Autodesk Inventor part; units mm, degrees
ref_plane "YZ Plane" through (0, 0, 0) normal (1, 0, 0) x (0, 1, 0)
ref_plane "XZ Plane" through (0, 0, 0) normal (0, 1, 0) x (-1, 0, 0)
ref_plane "XY Plane" through (0, 0, 0) normal (0, 0, 1) x (1, 0, 0)
sketch "Sketch1" plane through (0, 0, 0) normal (0, 1, 0) x (-1, 0, 0)
  line L0 (2.0728, 0) -> (87.1628, 0)
  line L1 (87.1628, 0) -> (87.1628, -50.165)
  line L2 (87.1628, -50.165) -> (2.0728, -50.165)
  line L3 (2.0728, -50.165) -> (2.0728, 0)
  line L4 (87.1628, -50.165) -> (2.0728, 0)
  point P0 (0, 0)
  dimension "d0" = 85.09
  dimension "d1" = 50.165
extrude "Extrusion1" add sketch "Sketch1" along normal blind 3.175 contours L0 L1 L4
sketch "Sketch2" plane through (0, 3.175, 0) normal (0, 1, 0) x (1, 0, 0)
  line L0 (-87.1628, 0) -> (-2.0728, 0)
  line L1 (-87.1628, 0) -> (-90.3378, 0)
  line L2 (-90.3378, 0) -> (-90.3378, 50.165)
  line L3 (-90.3378, 50.165) -> (-87.1628, 50.165)
  line L4 (-87.1628, 50.165) -> (-87.1628, 0)
  line L5 (-87.1628, 0) -> (-2.0728, 0)
  line L6 (-2.0728, 0) -> (-2.0728, -3.175)
  line L7 (-2.0728, -3.175) -> (-87.1628, -3.175)
  line L8 (-87.1628, -3.175) -> (-87.1628, 0)
  line L9 (-90.3378, 0) -> (-87.1628, 0)
  line L10 (-87.1628, 0) -> (-87.1628, -3.175)
  line L11 (-87.1628, -3.175) -> (-90.3378, -3.175)
  line L12 (-90.3378, -3.175) -> (-90.3378, 0)
  point P0 (0, 0)
  dimension "d4" = 3.175
  dimension "d5" = 3.175
extrude "Extrusion2" add sketch "Sketch2" along normal blind 34.7726 contours L1 L2 L3 L4 | L0 L6 L7 L8
sketch "Sketch3" plane through (0, 37.9476, 0) normal (0, 1, 0) x (1, 0, 0)
  line L0 (-87.1628, 0) -> (-90.3378, 0)
  line L1 (-90.3378, 0) -> (-90.3378, -3.175)
  line L2 (-90.3378, -3.175) -> (-87.1628, -3.175)
  line L3 (-87.1628, -3.175) -> (-87.1628, 0)
  point P0 (0, 0)
  dimension "d8" = 3.175
extrude "Extrusion3" add sketch "Sketch3" against normal blind 34.7726
sketch "Sketch4" plane through (0, 3.175, 0) normal (0, -1, 0) x (1, 0, 0)
  line L0 (-87.1628, 0) -> (-2.0728, 0)
  line L1 (-2.0728, 3.175) -> (-2.0728, 0)
  line L2 (-2.0728, 3.175) -> (-90.3378, 3.175)
  line L3 (-90.3378, -50.165) -> (-90.3378, 3.175)
  line L4 (-87.1628, -50.165) -> (-90.3378, -50.165)
  line L5 (-87.1628, -50.165) -> (-87.1628, 0)
  point P0 (0, 0)
extrude "Extrusion4" add sketch "Sketch4" along normal blind 3.175
fillet "Fillet1" radius 3.175 2 edges at (-46.2053, 0, 3.175) (-90.3378, 0, -23.495)
sketch "Sketch5" plane through (0, 0, 0) normal (0, -1, 0) x (1, 0, 0)
  line L0 (-87.0358, -0.127) -> (-90.3378, -0.127)
  line L1 (-90.3378, -0.127) -> (-90.3378, 3.175)
  line L2 (-90.3378, 3.175) -> (-87.0358, 3.175)
  line L3 (-87.0358, 3.175) -> (-87.0358, -0.127)
  line L4 (-90.3378, 0) -> (-90.3378, -50.165)
  line L5 (-2.0728, 3.175) -> (-87.1628, 3.175)
  point P0 (0, 0)
  dimension "d22" = 3.302
  dimension "d23" = 3.302
  dimension "d24" = 0
  dimension "d25" = 0
extrude "Extrusion5" cut sketch "Sketch5" against normal blind 127
chamfer "Chamfer4" distance 3.175 angle 45 4 edges at (-2.0728, 37.9476, 1.5875) (-88.7503, 37.9476, -50.165) (-88.7503, 37.9476, -0.127) (-87.0358, 37.9476, 1.5875)
sketch "Sketch6" plane through (-87.1628, 3.175, -0.127) normal (1, 0, 0) x (0, 0, -1)
  line L0 (50.038, 0) -> (50.038, 31.5976)
  line L1 (3.175, 34.7726) -> (46.863, 34.7726)
  circle A0 centre (38.608, 25.3746) radius 2.54
  circle A1 centre (38.608, 12.6746) radius 2.54
  circle A2 centre (25.908, 25.3746) radius 2.54
  circle A3 centre (25.908, 12.6746) radius 2.54
  circle A4 centre (13.208, 25.3746) radius 2.54
  circle A5 centre (13.208, 12.6746) radius 2.54
  point P0 (-0.127, -3.175)
  dimension "d43" = 25.4
  dimension "d32" = 5.08
  dimension "d34" = 11.43
  dimension "d35" = 9.398
  dimension "d36" = 5.08
  dimension "d37" = 12.7
  dimension "d40" = 12.7
extrude "Extrusion6" cut sketch "Sketch6" against normal blind 127
sketch "Sketch7" plane through (-2.0728, 3.175, 0) normal (0, 0, -1) x (-1, 0, 0)
  line L0 (3.175, 34.7726) -> (81.788, 34.7726)
  line L1 (84.963, 0) -> (0, 0)
  line L2 (84.963, 0) -> (84.963, 31.5976)
  circle A0 centre (78.613, 25.8826) radius 2.54
  circle A1 centre (47.752, 25.8826) radius 2.54
  circle A2 centre (16.891, 25.8826) radius 2.54
  circle A3 centre (78.613, 11.6586) radius 2.54
  circle A4 centre (47.752, 11.6586) radius 2.54
  circle A5 centre (16.891, 11.6586) radius 2.54
  point P0 (-2.0728, -3.175)
  dimension "d48" = 5.08
  dimension "d49" = 6.35
  dimension "d50" = 8.89
  dimension "d53" = 30.861
  dimension "d56" = 14.224
extrude "Extrusion7" cut sketch "Sketch7" against normal blind 127
sketch "Sketch8" plane through (0, 3.175, 0) normal (0, 1, 0) x (1, 0, 0)
  line L0 (-87.0358, 0) -> (-2.0728, 0)
  line L1 (-87.1628, 50.165) -> (-87.1628, 0.127)
  circle A0 centre (-74.412, 36.0934) radius 2.54
  line L2 (-87.1628, 50.165) -> (-90.3378, 50.165)
  circle A1 centre (-61.839, 36.0934) radius 2.54
  circle A2 centre (-49.266, 36.0934) radius 2.54
  circle A3 centre (-36.693, 36.0934) radius 2.54
  circle A4 centre (-74.412, 23.5204) radius 2.54
  circle A5 centre (-61.839, 23.5204) radius 2.54
  circle A6 centre (-49.266, 23.5204) radius 2.54
  circle A7 centre (-36.693, 23.5204) radius 2.54
  circle A8 centre (-74.412, 10.9474) radius 2.54
  circle A9 centre (-61.839, 10.9474) radius 2.54
  circle A10 centre (-49.266, 10.9474) radius 2.54
  circle A11 centre (-36.693, 10.9474) radius 2.54
  point P0 (0, 0)
  dimension "d61" = 5.08
  dimension "d63" = 12.7508
  dimension "d64" = 14.0716
  dimension "d67" = 12.573
  dimension "d70" = 12.573
extrude "Extrusion8" cut sketch "Sketch8" against normal blind 127 contours A0 | A4 | A5 | A8 | A9 | A10 | A11
properties part number "Chassis_BumperAttachment Bruh"
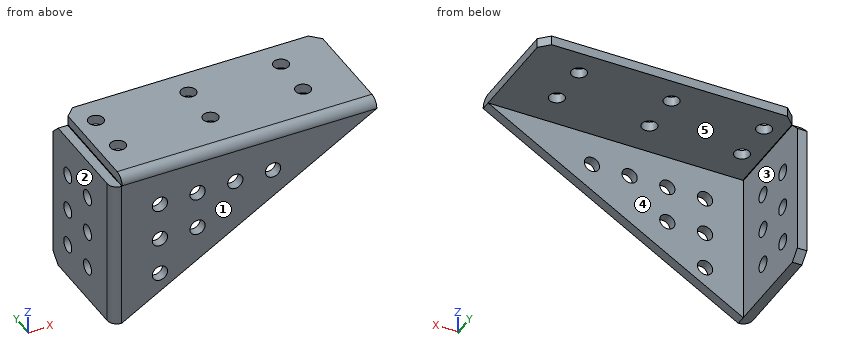
Input: part model. Units: mm. Frame: model coordinates. Face numbers are marked on the shaded views. A direction names the side the tool comes from. Give positions to 0.01 mm unless a question says otherwise; leave off trailing zeros. Order: outer loops, then holes, each group sorted by start corner. A loop starts at its lowest first (then second) coordinate and runs counter-clockwise, first axis right, second up. Notation, with made-up numbers: M 67.5,50 L 73.5,50 A30 ccw 73.5,88 Z; hole C 11.5,-0.5 d3. An arc over 180 degrees is marked long. Answer as a JSON object with one key per item and string values.
1. Reachability of the marked faces 1, 2, 3, 4 and 5 from +Z, -Z, +X, -X, +Y, -Y: full face, straight path, thin tool, end or side. Return the list, or none.
Result sheet:
{"face 1": "+Z, -Z, +X, -X, -Y", "face 2": "+Z, -Z, -X, +Y, -Y", "face 3": "+Z, -Z, +X, +Y", "face 4": "-Z, +X, +Y", "face 5": "-Z, +X, -X, +Y"}
2. Cut plane A-A, the plane y = 5.5. Output: boundary loops of the cut face in (x, z) (3 decimals), and give its area (3 significant figures).
Result sheet:
{"outline": "M -90.338,-50.165 L -87.163,-50.165 L -87.163,-0.127 L -90.338,-0.127 Z; M -87.036,0 L -2.073,0 L -2.073,3.175 L -87.036,3.175 Z", "area": "429 mm²"}
3. Cut plane C-C, the plane z = -35. Output: boundary loops of the cut face in (x, y) (3 decimals).
Result sheet:
{"outline": "M -90.338,3.175 A3.175 ccw -87.163,0 L -76.705,0 L -76.705,3.175 L -87.163,3.175 L -87.163,37.948 L -90.338,37.948 Z; M -72.119,0 L -61.44,0 L -61.44,3.175 L -72.119,3.175 Z"}
4. Ray query, line 1 (X direction, y = 11, z = -35); line 2 (Y direction, x = -61.5, z = -32.5) (3 decimals). Return the intervals inside material, ascending. Write a range as [from, to].
Result sheet:
{"line 1": "[-90.34, -87.16]", "line 2": "[0, 3.175]"}
5. Cut plane B-B, the plane x = -62. State how many separate pieces and enclosed holes the cut face has, and give its area (3 significant figures).
Result sheet:
{"separate pieces": "3", "enclosed holes": "0", "area": "198 mm²"}
6. Cut plane D-D, the plane x = -29. Output: boundary loops of the cut face in (y, z) (3 decimals).
Result sheet:
{"outline": "M 0,-15.875 L 3.175,-15.875 L 3.175,0 L 37.948,0 L 37.948,3.175 L 3.175,3.175 A3.175 ccw 0,0 Z"}
7. First-contact query: P1, Ø1, axis at x = -66, y = 7.5, coming from the -Z side; P2, Ø1.5, axis at y = 27, z = -16.5, coming from the +X side; P3, Ø15, axis at x = -64, z = -35, coming from the +Y side (3 decimals); P4, Ø4.5, axis at x = -74.41, z = -36.09, coming from the -Y side. Flat tips, straight axial feed; report the tip coordinate or a pass-through.
Result sheet:
{"P1": "z = 0", "P2": "x = -87.16", "P3": "y = 3.175", "P4": "through"}
